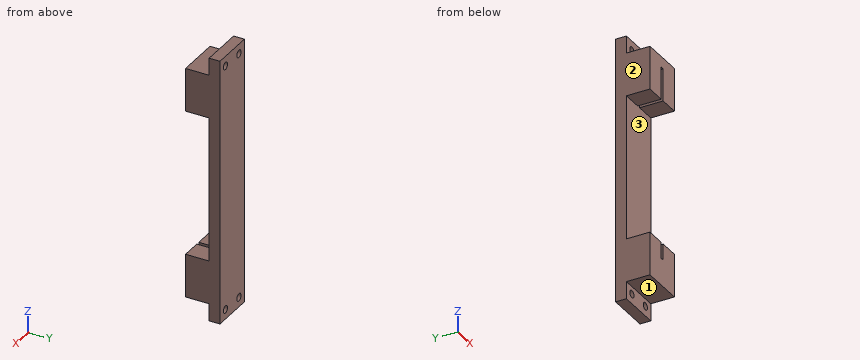
from build123d import *

# Parameters (mm, degrees)
SKETCH1_W            = 20
SKETCH1_H            = 28
BOSS_EXTRUDE1_DEPTH  = 5
SKETCH2_W            = 20
SKETCH2_H            = 20
BOSS_EXTRUDE2_DEPTH  = 10.9
SKETCH3_W            = 1.6
SKETCH3_H            = 15
CUT_EXTRUDE1_DEPTH   = 10.9
M3_CLEARANCE_HOLE1_D = 3.4
SKETCH6_W            = 20
SKETCH6_H            = 5
BOSS_EXTRUDE3_DEPTH  = 87
SKETCH7_W            = 20
SKETCH7_H            = 5
BOSS_EXTRUDE4_DEPTH  = 8
SKETCH8_W            = 20
SKETCH8_H            = 20
BOSS_EXTRUDE5_DEPTH  = 10.9
SKETCH9_W            = 1.6
SKETCH9_H            = 28.5
CUT_EXTRUDE2_DEPTH   = 10.9
M3_CLEARANCE_HOLE2_D = 3.4


with BuildPart() as part:
    # Sketch1 → Boss-Extrude1 (new body)
    with BuildSketch(Plane(origin=(0, 0, 0), x_dir=(1, 0, 0), z_dir=(0, 1, 0))):
        Rectangle(SKETCH1_W, SKETCH1_H)
    extrude(amount=BOSS_EXTRUDE1_DEPTH)

    # Sketch2 → Boss-Extrude2 (add)
    with BuildSketch(Plane(origin=(0, 0, 0), x_dir=(-1, 0, 0), z_dir=(0, -1, 0))):
        with Locations((0, 4)):
            Rectangle(SKETCH2_W, SKETCH2_H)
    extrude(amount=BOSS_EXTRUDE2_DEPTH)

    # Sketch3 → Cut-Extrude1 (cut)
    with BuildSketch(Plane(origin=(0, -10.9, 0), x_dir=(-1, 0, 0), z_dir=(0, -1, 0))):
        with Locations((0, 6.5)):
            Rectangle(SKETCH3_W, SKETCH3_H)
    extrude(amount=-CUT_EXTRUDE1_DEPTH, mode=Mode.SUBTRACT)

    # M3 Clearance Hole1 (through all)
    with Locations(Plane(origin=(0, 0, 0), x_dir=(-1, 0, 0), z_dir=(0, -1, 0))):
        with Locations((-5.5, -9.5), (5.5, -9.5)):
            Hole(M3_CLEARANCE_HOLE1_D / 2)

    # Sketch6 → Boss-Extrude3 (add)
    with BuildSketch(Plane(origin=(0, 0, -14), x_dir=(-1, 0, 0), z_dir=(0, 0, -1))):
        with Locations((0, 2.5)):
            Rectangle(SKETCH6_W, SKETCH6_H)
    extrude(amount=BOSS_EXTRUDE3_DEPTH)

    # Sketch7 → Boss-Extrude4 (add)
    with BuildSketch(Plane(origin=(0, 0, -101), x_dir=(-1, 0, 0), z_dir=(0, 0, -1))):
        with Locations((0, 2.5)):
            Rectangle(SKETCH7_W, SKETCH7_H)
    extrude(amount=BOSS_EXTRUDE4_DEPTH)

    # Sketch8 → Boss-Extrude5 (add)
    with BuildSketch(Plane(origin=(0, 0, 0), x_dir=(-1, 0, 0), z_dir=(0, -1, 0))):
        with Locations((0, 91)):
            Rectangle(SKETCH8_W, SKETCH8_H)
    extrude(amount=BOSS_EXTRUDE5_DEPTH)

    # Sketch9 → Cut-Extrude2 (cut)
    with BuildSketch(Plane(origin=(0, -10.9, 0), x_dir=(-1, 0, 0), z_dir=(0, -1, 0))):
        with Locations((0, 74.25)):
            Rectangle(SKETCH9_W, SKETCH9_H)
    extrude(amount=-CUT_EXTRUDE2_DEPTH, mode=Mode.SUBTRACT)

    # M3 Clearance Hole2 (through all)
    with Locations(Plane(origin=(0, 0, 0), x_dir=(-1, 0, 0), z_dir=(0, -1, 0))):
        with Locations((-5.5, 104.5), (5.5, 104.5)):
            Hole(M3_CLEARANCE_HOLE2_D / 2)


solid = part.part
Read the model definition and answer for the solid it produces. Units are mm, in the model's axes. Face numbers are marked on the shaded views. Coordinates: 2 decimals unless noted, no trailing zeros. Loops run counter-clockwise (first coordinate to the right, second up) from the corner with the lowest first, then second, coordinate; pieces in that order, holes last. Notation, with made-up numbers: (-19, -10) -> (27, -10) arc R13 ccw to (27, 5) -> close; hole circle Ø7 at (80.25, 23.5). An arc over 180 degrees is marked (long way). Write item = value, one per line. Start each with the question number.
1) The part is cut by section B-B, the plane x = 5.5. Determine the outline of the cut face in (y, z), plus the area to 3 significant figures.
2) The mould has two halves that part along Z. Classify the marked faces 1, 2 and 3: pulls with the +Z half, pulls with the -Z half, needs draft (parallel to the pull), parting line crosses it, or undercut.
3) Given P1, Ø3, axis at x = -7.5, y = -3.5, coming from the -Z side; P2, Ø4.5, axis at x = -5.5, z = 9.5, coming from the -Y side; P3, Ø7.5, axis at x = -3.5, y = -8, coming from the +Z side, each flat-ended and moving along its own axis, determine where each tip first touches the part or whether it passes through.
4) The part is cut by section A-A, the plane y = -7.25. Determine the outline of the cut face in (x, z).
5) Find the intervals of material crossed by L1, parallel to Z at x = 5.5, y = 2; L2, parallel to X at y = 3.7, z = 9.5; L3, parallel to Z at x = 0.5, y = -1.5, in increasing order. Write a range as from..to.
6) The part is cut by section C-C, the plane z = -51.5. Determine the outline of the cut face in (x, y).
Result:
q1.outline = (-10.9, -101) -> (0, -101) -> (0, -102.8) -> (5, -102.8) -> (5, 7.8) -> (0, 7.8) -> (0, 6) -> (-10.9, 6) -> (-10.9, -14) -> (0, -14) -> (0, -81) -> (-10.9, -81) -> close; (0, -109) -> (5, -109) -> (5, -106.2) -> (0, -106.2) -> close; (0, 11.2) -> (5, 11.2) -> (5, 14) -> (0, 14) -> close
q1.area = 1,020 mm²
q2.face_1 = pulls with the -Z half
q2.face_2 = needs draft
q2.face_3 = undercut
q3.P1 = -101
q3.P2 = 0
q3.P3 = 6
q4.outline = (-10, -101) -> (10, -101) -> (10, -81) -> (0.8, -81) -> (0.8, -88.5) -> (-0.8, -88.5) -> (-0.8, -81) -> (-10, -81) -> close; (-10, -14) -> (-0.8, -14) -> (-0.8, 1) -> (0.8, 1) -> (0.8, -14) -> (10, -14) -> (10, 6) -> (-10, 6) -> close
q5.L1 = -109..-106.2, -102.8..7.8, 11.2..14
q5.L2 = -10..-7.2, -3.8..3.8, 7.2..10
q5.L3 = -101..-88.5, 1..6
q6.outline = (-10, 0) -> (10, 0) -> (10, 5) -> (-10, 5) -> close
